For this review, use the dimensioned drawing (mm, ordinates from the lowest corner) and the shaded views. Give positions to 0.01 mm unless a question says otherwise; leave off trailing zeros. Order: outer loops, then holes, each group sorted by start corner. A loop starts at its lowest first (then second) coordinate and runs counter-clockwise, first axis right, second up. Notation, with made-up numbers: (30.25, -18) -> (89.25, -18) arc R35 ccw to (89.25, 14) -> close; hole circle Ø2 at (87.5, 20.25). An arc over 180 degrees is marked (long way). Return JSON: item names as keys, results as strings.
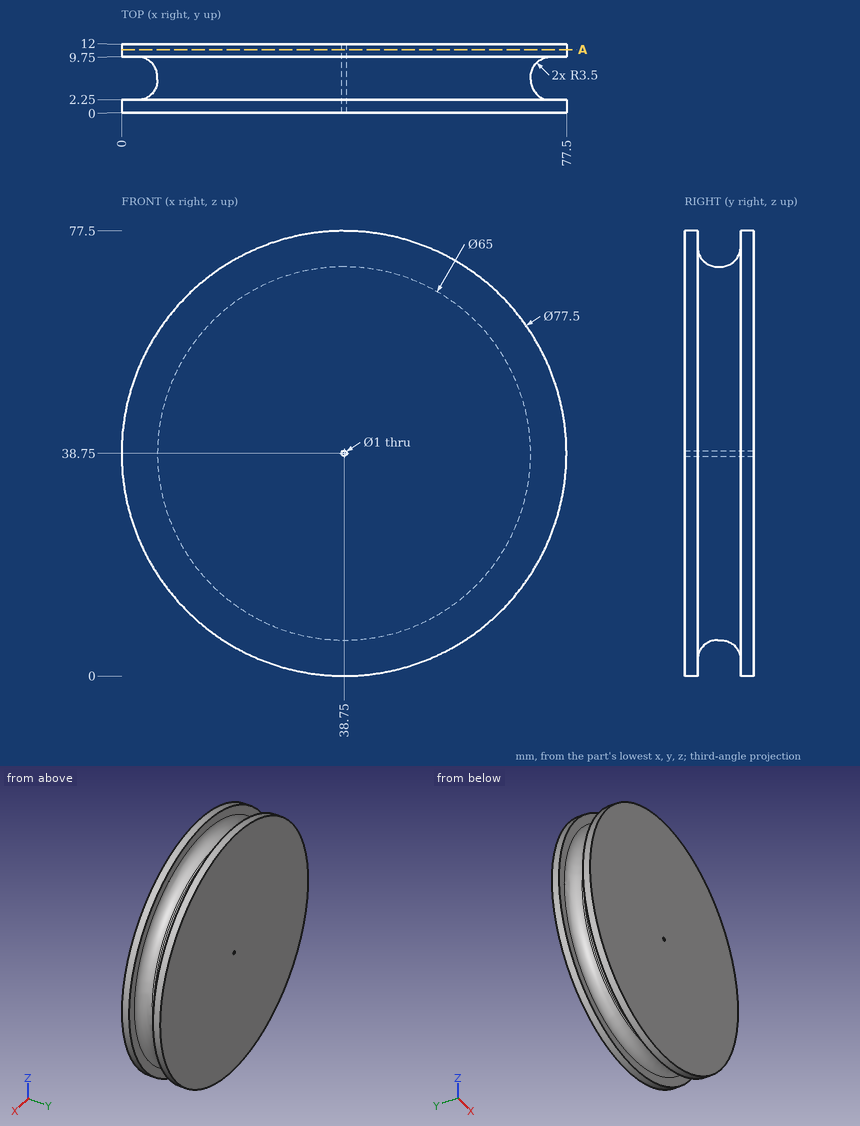
Item 1: Wall thickness on L1, parallel to X at y = 6.5, z = 38.75; L2, parallel to Y at x = 23.5, z = 6; L3, parallel to Y at x = 54.5, z = 8.5: over which ranges is each line inside the solid? List them lowest first. Write a range as [from, to].
Result set:
{"L1": "x = [6.24, 38.25], [39.25, 71.26]", "L2": "y = [0, 2.25], [9.75, 12]", "L3": "y = [0, 2.81], [9.19, 12]"}
Item 2: For pin 1 (6 mm diameter, centred on y = 8.5, z = 27.5, fed in from +X); pin 2 (2 mm diameter, centred on y = 10, z = 42.5, fed in from -X); pin 3 (3 mm diameter, centred on x = 12, y = 4.5, fed in from -Z), all flat-tipped, find the tip position at first contact; note any pin that passes through.
Result set:
{"pin 1": "stops at x = 76.55", "pin 2": "stops at x = 0.1", "pin 3": "stops at z = 17.44"}
Item 3: Add section A-A (y = 11). Give the boundary of the cut face in (x, z).
Result set:
{"outline": "circle Ø77.5 at (38.75, 38.75); hole circle Ø1 at (38.75, 38.75)"}
